Can you work these out from the model? Positions are in its coordinate system, mm. Face numbers are marked on the shaded views. Coordinates: 2 decimals unless noted, no trailing zeros. Loops run counter-clockwise (first coordinate to the right, second up) from the corner with the lowest first, then second, coordinate; pieces in that order, holes last. Notation, with made-up numbers: (-3.75, 4.5) -> (40.25, 4.5) arc R27 cw to (40.25, 30.5) -> close; hole circle Ø7 at (-35.75, 24.25). An arc over 180 degrees is marked (long way). Use one line per item in the form item = value. Start each with the question number.
(1) I need wall thicknesses on line 1 (X direction, y = 3.5, z = 0); line 2 (Z direction, x = 4, y = 1); line 3 (X direction, y = 0.5, z = -1.25). Which ranges of each line are inside material? Lowest first, please. Write a range as [from, to].
(2) I'm going to push flat-ended pins straight in: pin 1 (2 mm diameter, centred on x = 2.5, y = 4.5, fed in from +Z); pin 2 (1.5 mm diameter, centred on y = 6.5, z = 2.5, fed in from -X). Where does each tip first touch, or does it pass through?
(3) Imagine slicing it at B-B (y = 6.25). List the corners of the cut face in (x, z) for me, plus the area to 3 significant figures.
(4) Imagine slicing it at C-C (x = 0). List the corners of the cut face in (y, z) for me.
(5) Imagine slicing it at D-D (y = 9.25). List the corners of the cut face in (x, z) for me, plus the area to 3 significant figures.
(6) Imagine slicing it at A-A (z = 0). List the corners of the cut face in (x, y) for me.
(7) Thinking about a two-plate mould opening in Z: for the marked faces 1, 2 and 3, which applies, released by +Z, released by -Z, zero draft, split by the parting line, or undercut?
```python
from build123d import *

# Parameters (mm, degrees)
SKETCH_1_R          = 5
EXTRUDE_1_DEPTH     = 10
SKETCH_2_R          = 1.95
CUT_EXTRUDE_1_DEPTH = 8.6
FILLET_1_R          = 1


with BuildPart() as part:
    # Эскиз1 → Бобышка-Вытянуть1 (new body)
    with BuildSketch(Plane(origin=(0, 0, 0), x_dir=(1, 0, 0), z_dir=(0, 1, 0))):
        with Locations(Location((0, 0, 0), (0, 0, 270))):
            Circle(SKETCH_1_R)
    extrude(amount=EXTRUDE_1_DEPTH)

    # Эскиз2 → Вырез-Вытянуть1 (cut)
    with BuildSketch(Plane(origin=(0, 10, 0), x_dir=(1, 0, 0), z_dir=(0, 1, 0))):
        with Locations(Location((0, 0, 0), (0, 0, 270))):
            Circle(SKETCH_2_R)
    extrude(amount=-CUT_EXTRUDE_1_DEPTH, mode=Mode.SUBTRACT)

    # Скругление1
    fillet_1_edges = [part.edges().sort_by_distance(p)[0] for p in [
        (0, 10, -1.95),
    ]]
    fillet(fillet_1_edges, radius=FILLET_1_R)


solid = part.part
```
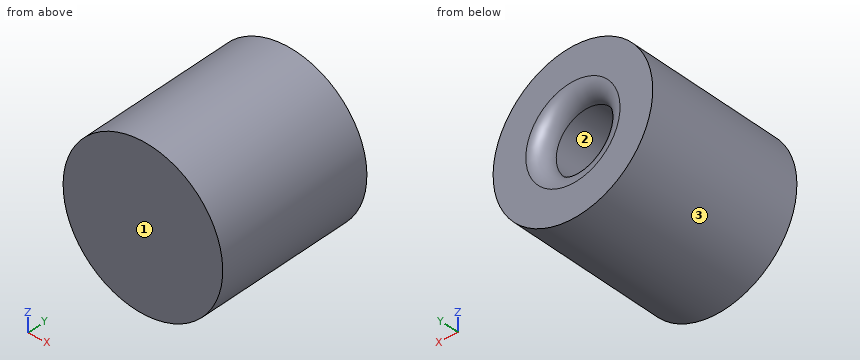
Worked out:
q1.line_1 = [-5, -1.95], [1.95, 5]
q1.line_2 = [-3, 3]
q1.line_3 = [-4.84, 4.84]
q2.pin_1 = 4.77
q2.pin_2 = -4.68
q3.outline = circle Ø10 at (0, 0); hole circle Ø3.9 at (0, 0)
q3.area = 66.6 mm2
q4.outline = (0, -5) -> (10, -5) -> (10, -2.95) arc R1 ccw to (9, -1.95) -> (1.4, -1.95) -> (1.4, 1.95) -> (9, 1.95) arc R1 ccw to (10, 2.95) -> (10, 5) -> (0, 5) -> close
q5.outline = circle Ø10 at (0, 0); hole circle Ø3.96 at (0, 0)
q5.area = 66.2 mm2
q6.outline = (-5, 0) -> (5, 0) -> (5, 10) -> (2.95, 10) arc R1 ccw to (1.95, 9) -> (1.95, 1.4) -> (-1.95, 1.4) -> (-1.95, 9) arc R1 ccw to (-2.95, 10) -> (-5, 10) -> close
q7.face_1 = zero draft
q7.face_2 = undercut
q7.face_3 = split by the parting line
